from build123d import *

# Parameters (mm, degrees)
BOSS_EXTRUDE1_DEPTH = 25.875
FILLET1_R           = 2
SKETCH2_R           = 7.9375
BOSS_EXTRUDE2_DEPTH = 18.3
SKETCH3_W           = 25.875
SKETCH3_H           = 34.7
BOSS_EXTRUDE3_DEPTH = 2


with BuildPart() as part:
    # Sketch1 → Boss-Extrude1 (new body)
    with BuildSketch(Plane(origin=(0, 0, 0), x_dir=(0, 0, -1), z_dir=(1, 0, 0))):
        Polygon((-26.5, -27.5), (-26.5, -5.5), (-23.5, -5.5), (-23.5, -15.5), (-20.5, -15.5), (-20.5, -12.5), (-17.5, -12.5), (-17.5, -17.5), (-12, -17.5), (-12, -20.5), (-15, -20.5), (-15, -23.5), (0, -23.5), (0, -27.5), align=None)
    extrude(amount=BOSS_EXTRUDE1_DEPTH)

    # Fillet1
    fillet1_edges = [part.edges().sort_by_distance(p)[0] for p in [
        (12.9375, -12.5, 17.5),
        (12.9375, -17.5, 12),
    ]]
    fillet(fillet1_edges, radius=FILLET1_R)

    # Mirror1: part across plane


with BuildPart() as part_1:
    add(part.part)
    add(part.part.mirror(Plane(origin=(25.875, -23.5, 0), x_dir=(1, 0, 0), z_dir=(0, 0, 1))))

    # Sketch2 → Boss-Extrude2 (add)
    with BuildSketch(Plane(origin=(0, 0, 26.5), x_dir=(-1, 0, 0), z_dir=(0, 0, -1))):
        with BuildLine():
            Line((-25.875, -27.5), (-25.875, -40.4375))
            ThreePointArc((-25.875, -40.4375), (-12.9375, -53.375), (0, -40.4375))
            Line((0, -40.4375), (0, -27.5))
            Line((0, -27.5), (0, -23.5))
            Line((0, -23.5), (-25.875, -23.5))
            Line((-25.875, -23.5), (-25.875, -27.5))
        make_face()
        with Locations((-12.9375, -40.4375)):
            Circle(SKETCH2_R, mode=Mode.SUBTRACT)
    extrude(amount=BOSS_EXTRUDE2_DEPTH)

    # Sketch3 → Boss-Extrude3 (add)
    with BuildSketch(Plane.XZ.offset(27.5)):
        with Locations((12.9375, -9.15)):
            Rectangle(SKETCH3_W, SKETCH3_H)
    extrude(amount=BOSS_EXTRUDE3_DEPTH)


solid = part_1.part
Work out the finished part from the listing and answer in its coordinate system (mm). A direction names the side the tool comes from. Round coordinates to 2 decimals unless told otherwise and drop trailing zeros. Write each loop counter-clockwise with the first axis right and the second up, starting at its lowest first coordinate (ties: lowest second). Pieces come first, ordered by that corner, then holes. Notation, with made-up numbers: (81.5, 28.5) -> (137.5, 28.5) arc R18 ccw to (137.5, 56.5) -> close; hole circle Ø2 at (-5, 74). An arc over 180 degrees is marked (long way). Write each question's results on one line, items separated by ' | '.
Item 1: A cutting plane is placed at A-A, the plane z = 13. Determine the outline of the cut face in (x, y) (1 decimal).
Result set:
outline: (0, -40.4) arc R12.9 ccw to (25.9, -40.4) -> (25.9, -23.5) -> (0, -23.5) -> close; (0, -20.5) -> (25.9, -20.5) -> (25.9, -17.8) -> (0, -17.8) -> close; hole circle Ø15.9 at (12.9, -40.4)
Item 2: Find the intervals of material crossed by line 1 along Z through (x, y) = (14.5, -20); line 2 along Z through (x, y) = (4.5, -10); line 3 along Y through (x, z) = (7.75, 9), in increasing order. Write a range as [from, to].
Result set:
line 1: [-26.5, -12], [12, 26.5] | line 2: [-26.5, -23.5], [23.5, 26.5] | line 3: [-52.29, -46.45], [-34.43, -23.5]
Item 3: A cutting plane is placed at B-B, the plane y = -39. Determine the outline of the cut face in (x, z) (3 decimals), plus the area to 3 significant figures.
Result set:
outline: (0, 8.2) -> (5.131, 8.2) -> (5.131, 26.5) -> (0, 26.5) -> close; (20.744, 8.2) -> (25.875, 8.2) -> (25.875, 26.5) -> (20.744, 26.5) -> close | area: 188 mm^2
Item 4: Flat-ended cylindrical pins translate along their axes: P1, Ø0.8, axis at x = 10, z = -20, coming from the +Y side; P2, Ø4, axis at x = 21, z = -11, coming from the -Y side; P3, Ø10, axis at x = 10, z = 19, coming from the +Y side; P4, Ø8, axis at x = 12.5, z = 1.5, coming from the +Y side. Find the tip coordinate at first contact, or state that the pin passes through.
Result set:
P1: y = -12.5 | P2: y = -29.5 | P3: y = -5.5 | P4: y = -23.5
Item 5: A cutting plane is placed at D-D, the plane y = -47. Determine the outline of the cut face in (x, z), plus the area to 3 significant figures.
Result set:
outline: (1.79, 8.2) -> (8.47, 8.2) -> (8.47, 26.5) -> (1.79, 26.5) -> close; (17.4, 8.2) -> (24.09, 8.2) -> (24.09, 26.5) -> (17.4, 26.5) -> close | area: 245 mm^2
Item 6: The mould has two halves that part along X. Classify faces 5 (the face through (14.658, -48.186, 17.478)), 6 (the face through (7, -47, 8.2)), 7 (the face through (13.22, -53.37, 17.48)), 8 (the face through (0, -27, 0)): +X half, -X half, draft (parallel to the pull), parting line (faces both ways), or undercut.
Result set:
face 5: undercut | face 6: draft | face 7: parting line | face 8: -X half
Item 7: Which of the six approach directions +Z, -Z, +X, -X, +Y, -Y give full straight-line access (tool end or side, diameter ignored) to faces 1 (the face through (13, -29.5, -9)), 2 (the face through (13, -20.5, -13)), 3 (the face through (13, -5.5, 25)), 4 (the face through (13.12, -13.07, 18.1))?
Result set:
face 1: -Z, +X, -X, -Y | face 2: +X, -X | face 3: +Z, -Z, +X, -X, +Y | face 4: +X, -X, +Y
